from build123d import *

# Parameters (mm, degrees)
SKETCH1_W             = 72
SKETCH1_H             = 125
BOSS_EXTRUDE1_DEPTH   = 5
SKETCH2_R             = 1.5
CUT_EXTRUDE6_DEPTH    = 5
BOSS_EXTRUDE2_DEPTH   = 60
BOSS_EXTRUDE3_START   = -30.5
BOSS_EXTRUDE3_DEPTH   = 1.5
BOSS_EXTRUDE3_START_2 = 29
BOSS_EXTRUDE3_2_DEPTH = 1.5
BOSS_EXTRUDE3_START_3 = -29
BOSS_EXTRUDE3_3_DEPTH = 5
BOSS_EXTRUDE3_START_4 = 24
BOSS_EXTRUDE3_4_DEPTH = 5
SKETCH5_W             = 1
SKETCH5_H             = 65
SKETCH5_W_2           = 4
CUT_EXTRUDE7_DEPTH    = 158


# Read off the part's stored shape, not the designer's step: Boss-Extrude3
with BuildPart() as part:
    # Sketch1 → Boss-Extrude1 (new body)
    with BuildSketch(Plane(origin=(0, 0, 0), x_dir=(-1, 0, 0), z_dir=(0, 0, 1))):
        with Locations((0, -8.5305)):
            Rectangle(SKETCH1_W, SKETCH1_H)
    extrude(amount=BOSS_EXTRUDE1_DEPTH)

    # Sketch2 → Cut-Extrude6 (cut)
    with BuildSketch(Plane(origin=(0, 0, 0), x_dir=(-1, 0, 0), z_dir=(0, 0, 1))):
        with Locations(Location((30.5, -67.5305, 0), (0, 0, 180))):
            Circle(SKETCH2_R)
        with Locations(Location((-30.5, -67.5305, 0), (0, 0, 180))):
            Circle(SKETCH2_R)
        with Locations(Location((30.5, 25.4695, 0), (0, 0, 180))):
            Circle(SKETCH2_R)
        with Locations(Location((-30.5, 25.4695, 0), (0, 0, 180))):
            Circle(SKETCH2_R)
        with Locations(Location((0, -21.0305, 0), (0, 0, 180))):
            Circle(SKETCH2_R)
    extrude(amount=CUT_EXTRUDE6_DEPTH, mode=Mode.SUBTRACT)

    # Sketch3 → Boss-Extrude2 (add)
    with BuildSketch(Plane.XY.offset(5)):
        Polygon((-30.5, -53.9695), (-30.5, 65.5305), (30.5, 65.5305), (30.5, -53.9695), (36, -53.9695), (36, 71.0305), (-36, 71.0305), (-36, -53.9695), align=None)
    extrude(amount=BOSS_EXTRUDE2_DEPTH)

    # Boss-Extrude3 outline → Boss-Extrude3 (add)
    with BuildSketch(Plane.YZ.offset(BOSS_EXTRUDE3_START)):
        Polygon((-53.9695, 19), (25.428445475, 5), (65.5305, 5), (65.5305, 38.928925805), (-53.9695, 60), align=None)
    extrude(amount=BOSS_EXTRUDE3_DEPTH)

    # Boss-Extrude3 2 outline → Boss-Extrude3 2 (add)
    with BuildSketch(Plane.YZ.offset(BOSS_EXTRUDE3_START_2)):
        Polygon((-53.9695, 19), (25.428445475, 5), (65.5305, 5), (65.5305, 38.928925805), (-53.9695, 60), align=None)
    extrude(amount=BOSS_EXTRUDE3_2_DEPTH)

    # Boss-Extrude3 3 outline → Boss-Extrude3 3 (add)
    with BuildSketch(Plane.YZ.offset(BOSS_EXTRUDE3_START_3)):
        Polygon((-53.9695, 24), (-53.9695, 19), (25.428445475, 5), (53.784854573, 5), align=None)
        Polygon((-53.9695, 60), (-53.9695, 55), (65.5305, 33.928925805), (65.5305, 38.928925805), align=None)
    extrude(amount=BOSS_EXTRUDE3_3_DEPTH)

    # Boss-Extrude3 4 outline → Boss-Extrude3 4 (add)
    with BuildSketch(Plane.YZ.offset(BOSS_EXTRUDE3_START_4)):
        Polygon((-53.9695, 24), (-53.9695, 19), (25.428445475, 5), (53.784854573, 5), align=None)
        Polygon((-53.9695, 60), (-53.9695, 55), (65.5305, 33.928925805), (65.5305, 38.928925805), align=None)
    extrude(amount=BOSS_EXTRUDE3_4_DEPTH)

    # Sketch5 → Cut-Extrude7 (cut)
    with BuildSketch(Plane(origin=(0, 71.0305, 0), x_dir=(1, 0, 0), z_dir=(0, 1, 0))):
        with Locations((-35.5, -32.5)):
            Rectangle(SKETCH5_W, SKETCH5_H)
        with Locations((-38, -32.5)):
            Rectangle(SKETCH5_W_2, SKETCH5_H)
        with Locations((38, -32.5)):
            Rectangle(SKETCH5_W_2, SKETCH5_H)
        with Locations((35.5, -32.5)):
            Rectangle(SKETCH5_W, SKETCH5_H)
    extrude(amount=-CUT_EXTRUDE7_DEPTH, mode=Mode.SUBTRACT)


solid = part.part
Can you work these out from the model? Positions are in its coordinate system, mm. A direction names the side the tool comes from. Coordinates: 2 decimals unless noted, no trailing zeros. Loops run counter-clockwise (first coordinate to the right, second up) from the corner with the lowest first, then second, coordinate; pieces in that order, holes last. Notation, with made-up numbers: M 9.5,-28 L 15.5,-28 A22 ccw 15.5,11 Z; hole C 40,46 d9. An arc over 180 degrees is marked long. Return JSON: item names as keys, results as strings. Group by question number.
Item 1: Imagine slicing it at D-D (y = 37.5). Please give me the cut outline in (x, z).
Item 2: On a 3-axis mill with a long thin cutter (end or side, diameter ignored), from which of +Z, -Z, +X, -X, +Y, -Y can I reach the whole of each face in a straight line? I mean faces 1 (the flat face through (-24, 6, 47)), 2 (the flat face through (30.5, 20, 55)), 3 (the flat face through (30, 68, 5)). Say none if no direction works.
Item 3: If I drill on L1, parallel to Y at x = -30.5, z = 3.15; L2, parallel to X at y = -16, z = 17; L3, parallel to X at y = 49, z = 14.5, over which ranges is the centre line in solid material (lowest first)? Write a range as from..to.
Item 4: Thinking about a two-plate mould opening in Y: for faces 4 (the cylindrical face through (-31.69, -26.38, 2.46)), 5 (the flat face through (-26.535, 4.944, 44.612)), 6 (the flat face through (24, 6, 47)), which applies, released by +Y, released by -Y, zero draft, split by the parting line, or undercut?
Item 5: I'm going to push flat-ended pins straight in: pin 1 Ø3.5 at (x, y) = (-31, 68) entering from -Z; pin 2 Ø8 at (x, z) = (-18.5, 22) entering from -Y; pin 3 Ø0.9 at (x, y) = (30, 67) entering from -Z. Where does each tip first touch, or does it pass through?
Item 6: Imagine slicing it at B-B (x = 0). Please give me the cut outline in (y, z).
Item 7: Imagine slicing it at A-A (z = 26.5). Please give me the cut outline in (x, y), and give its area (3 significant figures).
Item 8: Imagine slicing it at C-C (x = 25.5). Please give me the cut outline in (y, z), and give its area (3 significant figures).
Verdict:
{
 "1": {"outline": "M -35,0 L 35,0 L 35,65 L 30.5,65 L 30.5,43.87 L 24,43.87 L 24,38.87 L 29,38.87 L 29,7.87 L 24,7.87 L 24,5 L -24,5 L -24,7.87 L -29,7.87 L -29,38.87 L -24,38.87 L -24,43.87 L -30.5,43.87 L -30.5,65 L -35,65 Z"},
 "2": {"face 1": "+Z, -Y", "face 2": "+Z", "face 3": "-Z"},
 "3": {"L1": "y = -53.97..-26.97, -23.97..66.03, 69.03..71.03", "L2": "x = -35..-24, 24..35", "L3": "x = -35..-29, 29..35"},
 "4": {"face 4": "undercut", "face 5": "released by -Y", "face 6": "zero draft"},
 "5": {"pin 1": "stops at z = 0", "pin 2": "stops at y = 65.53", "pin 3": "stops at z = 5"},
 "6": {"outline": "M -53.97,0 L 19.53,0 L 19.53,5 L -53.97,5 Z; M 22.53,0 L 71.03,0 L 71.03,65 L 65.53,65 L 65.53,5 L 22.53,5 Z"},
 "7": {"outline": "M -35,-53.97 L -29,-53.97 L -29,65.53 L 29,65.53 L 29,-53.97 L 35,-53.97 L 35,71.03 L -35,71.03 Z", "area": "1,820 mm^2"},
 "8": {"outline": "M -53.97,0 L 71.03,0 L 71.03,65 L 65.53,65 L 65.53,38.93 L -53.97,60 L -53.97,55 L 65.53,33.93 L 65.53,5 L 53.78,5 L -53.97,24 L -53.97,19 L 25.43,5 L -53.97,5 Z", "area": "2,020 mm^2"}
}
